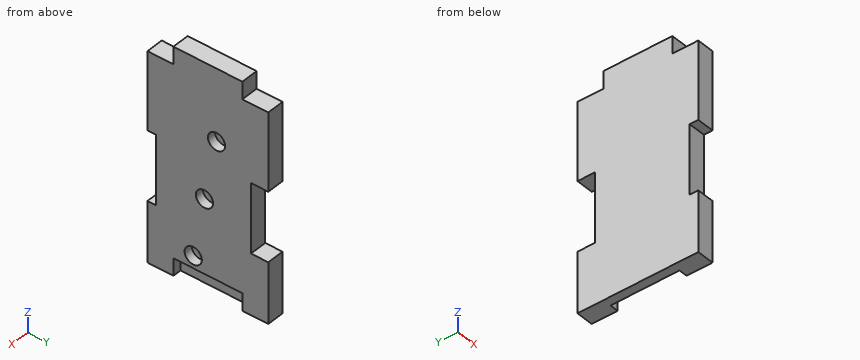
```python
from build123d import *

# Parameters (mm, degrees)
BOSS_EXTRUDE1_DEPTH = 5
SKETCH5_R           = 5
CUT_EXTRUDE4_DEPTH  = 5
SKETCH2_R           = 5
CUT_EXTRUDE5_DEPTH  = 5
BOSS_EXTRUDE2_DEPTH = 5
SKETCH7_W           = 10
SKETCH7_H           = 40
CUT_EXTRUDE6_DEPTH  = 5


with BuildPart() as part:
    # Sketch1 → Boss-Extrude1 (new body)
    with BuildSketch(Plane(origin=(0, 0, 0), x_dir=(0, 0, -1), z_dir=(1, 0, 0))):
        Polygon((-75, 70), (-120, 70), (-120, 55), (-130, 55), (-130, 15), (-120, 15), (-120, 0), (-75, 0), (-75, 5), (-35, 5), (-35, 0), (-10, 0), (0, 0), (0, 15), (0, 55), (0, 70), (-10, 70), (-35, 70), (-35, 60), (-75, 60), align=None)
    extrude(amount=BOSS_EXTRUDE1_DEPTH)

    # Sketch5 → Cut-Extrude4 (cut)
    with BuildSketch(Plane.ZY):
        with Locations((17.111667647, 26.5)):
            Circle(SKETCH5_R)
        with Locations((52.52, 33)):
            Circle(SKETCH5_R)
    extrude(amount=-CUT_EXTRUDE4_DEPTH, mode=Mode.SUBTRACT)

    # Sketch2 → Cut-Extrude5 (cut)
    with BuildSketch(Plane(origin=(5, 0, 0), x_dir=(0, 0, -1), z_dir=(1, 0, 0))):
        with Locations((-88.52, 40)):
            Circle(SKETCH2_R)
    extrude(amount=-CUT_EXTRUDE5_DEPTH, mode=Mode.SUBTRACT)

    # Sketch6 → Boss-Extrude2 (add)
    with BuildSketch(Plane.ZY):
        Polygon((35, 0), (35, 5), (75, 5), (75, 0), (120, 0), (120, 15), (130, 15), (130, 55), (120, 55), (120, 70), (75, 70), (75, 60), (35, 60), (35, 70), (0, 70), (0, 0), align=None)
    extrude(amount=BOSS_EXTRUDE2_DEPTH)

    # Sketch7 → Cut-Extrude6 (cut)
    with BuildSketch(Plane(origin=(5, 0, 0), x_dir=(0, 0, -1), z_dir=(1, 0, 0))):
        with Locations((-5, 35)):
            Rectangle(SKETCH7_W, SKETCH7_H)
    extrude(amount=-CUT_EXTRUDE6_DEPTH, mode=Mode.SUBTRACT)


solid = part.part
```
The listing builds one solid part. Answer for the finished solid, in the listing's coordinates (mm). Round coordinates to 2 decimals unless told otherwise and drop trailing zeros. Order: outer loops, then holes, each group sorted by start corner. A loop starts at its lowest first (then second) coordinate and runs counter-clockwise, first axis right, second up. Notation, with made-up numbers: (4.25, 5) - (50.25, 5) arc R31 ccw to (50.25, 44) - close; hole circle Ø4 at (-33.5, 13). An arc over 180 degrees is marked (long way). Put each result on its own line as item: value. Start each with the question number.
(1) Given P1, Ø3, axis at y = 25, z = 19, coming from the +X side; P2, Ø3, axis at x = 2.5, y = 62.5, coming from the +Z side; P3, Ø1.5, axis at x = -0.5, z = 59, coming from the +Y side, each flat-ended and moving along its own axis, determine where each tip first touches the part or whether it passes through.
(2) Find section D-D (x = -1.75). Give the vertices of the cut face in (y, z).
(3) Find section B-B (z = 52.52). Give the vertices of the cut face in (x, y), plus the area to 3 significant figures.
(4) Find section C-C (y = 40). Give the vertices of the cut face in (x, z).
(5) Find section A-A (x = 3.5). Give the vertices of the cut face in (y, z), plus the area to 3 significant figures.
(6) Straight lines are drawn through the part: probe 1 along Y at (x, z) = (2.9, 52.52); probe 2 along Z at (x, y) = (0.5, 63.5); probe 3 along Y at (x, z) = (2.85, 88.52). For each, find the intervals that lie inside material, in ascending order. Write a range as from..to.
Reply:
1. P1: x = 0
1. P2: z = 120
1. P3: y = 60
2. outline: (0, 0) - (70, 0) - (70, 35) - (60, 35) - (60, 75) - (70, 75) - (70, 120) - (55, 120) - (55, 130) - (15, 130) - (15, 120) - (0, 120) - (0, 75) - (5, 75) - (5, 35) - (0, 35) - close
3. outline: (-5, 5) - (5, 5) - (5, 28) - (0, 28) - (0, 38) - (5, 38) - (5, 60) - (-5, 60) - close
3. area: 500 mm^2
4. outline: (-5, 0) - (0, 0) - (0, 10) - (5, 10) - (5, 83.52) - (0, 83.52) - (0, 93.52) - (5, 93.52) - (5, 130) - (-5, 130) - close
5. outline: (0, 0) - (15, 0) - (15, 10) - (55, 10) - (55, 0) - (70, 0) - (70, 35) - (60, 35) - (60, 75) - (70, 75) - (70, 120) - (55, 120) - (55, 130) - (15, 130) - (15, 120) - (0, 120) - (0, 75) - (5, 75) - (5, 35) - (0, 35) - close; hole circle Ø10 at (26.5, 17.11); hole circle Ø10 at (33, 52.52); hole circle Ø10 at (40, 88.52)
5. area: 7,560 mm^2
6. probe 1: 5..28, 38..60
6. probe 2: 0..35, 75..120
6. probe 3: 0..35, 45..70
